Autodesk Inventor part; units mm, degrees
ref_plane "YZ Plane" through (0, 0, 0) normal (1, 0, 0) x (0, 1, 0)
ref_plane "XZ Plane" through (0, 0, 0) normal (0, 1, 0) x (-1, 0, 0)
ref_plane "XY Plane" through (0, 0, 0) normal (0, 0, 1) x (1, 0, 0)
sketch "Sketch1" plane through (0, 0, 0) normal (1, 0, 0) x (0, 1, 0)
  circle A0 centre (0, 0) radius 3
  dimension "d0" = 6
extrude "Extrusion1" add sketch "Sketch1" along normal mid plane 18
sketch "Sketch2" plane through (-9, 0, 0) normal (-1, 0, 0) x (0, 0, 1)
  circle A0 centre (0, 0) radius 4.5
  dimension "d3" = 9
extrude "Extrusion2" add sketch "Sketch2" along normal blind 1
sketch "Sketch3" plane through (9, 0, 0) normal (1, 0, 0) x (0, 0, -1)
  circle A0 centre (0, 0) radius 3.25
  dimension "d6" = 6.5
extrude "Extrusion3" add sketch "Sketch3" along normal blind 1
sketch "Sketch4" plane through (10, 0, 0) normal (1, 0, 0) x (0, 0, -1)
  circle A0 centre (0, 0) radius 3.25
  line L0 (-3.1282, 0.8815) -> (3.1282, 0.8815)
  line L1 (-3.25, 0) -> (3.25, 0)
  line L2 (-3.1282, -0.8815) -> (3.1282, -0.8815)
  arc A1 (-3.1282, 0.8815) -> (-3.1282, -0.8815) centre (0, 0) ccw
  arc A2 (3.1282, -0.8815) -> (3.1282, 0.8815) centre (0, 0) ccw
extrude "Extrusion4" cut sketch "Sketch4" against normal blind 19 contours L1 A0 L0 | A0 L2 L1
fillet "Fillet1" radius 2 2 edges at (10, 3.25, 0) (10, -3.25, 0)
properties part number "OsovinaZaPrednjiKotač_v.1.0"
The model under review builds one solid part; all positions refer to its coordinate system, in mm. A direction names the side the tool comes from. Round coordinates to 2 decimals unless told otherwise and drop trailing zeros. Order: outer loops, then holes, each group sorted by start corner. A loop starts at its lowest first (then second) coordinate and runs counter-clockwise, first axis right, second up. Notation, with made-up numbers: (-40, 53) -> (-5, 53) arc R21 ccw to (-5, 72) -> close; hole circle Ø10 at (54, -9). An arc over 180 degrees is marked (long way). One line per item, written item: value. Start each with the question number.
Q1. Take a section at A-A (x = 5.5). Write out the cut boundary in (y, z), and give its area (3 significant figures).
Q2. Clearance check with flat-ended pins moving along their axes: pin 1 Ø5 at (x, z) = (4.5, 1.5) entering from +Y; pin 2 Ø1.5 at (y, z) = (-2, 1.5) entering from +X; pin 3 Ø1.5 at (x, y) = (3.5, 3.5) entering from +Z. State where each tip first meets the part, or that it passes through.
Q3. Take a section at B-B (y = 4). Write out the cut boundary in (x, z), and give its area (3 significant figures).
Q4. Mouldability with a two-part tool opening along X and no side actions: class faces 4 (the face through (-10, 0, 0)), 5 (the face through (0, -3, 0)), 6 (the face through (0, 3, 0)), 7 (the face through (1, -0.882, 0)) as released by +X, released by -X, zero draft, split by the parting line, or undercut.
Q5. Wall thickness on line 1 (X direction, y = 4, z = 0); line 2 (Y direction, x = 7.75, z = 0.75); line 3 (Y direction, x = -4.5, z = 1.75): over which ranges is each line inside the solid? List them lowest first.
Q6. Machinability: for faces 1 (the face through (-9, 0, 0)), 2 (the face through (1, 0.882, 0)), 3 (the face through (-9.49, -4.46, -0.59)), which of the approach directions +Z, -Z, +X, -X, +Y, -Y give a long, thin tool a straight path to every point of the face, cutting with its end or side? Answer none if there is none.
Reported:
1. outline: (-0.88, -2.87) -> (-0.88, 2.87) arc R3 ccw to start; (0.88, -2.87) arc R3 ccw to (0.88, 2.87) -> close
1. area: 17.9 mm2
2. pin 1: stops at y = 3
2. pin 2: stops at x = 9.99
2. pin 3: stops at z = 1.2
3. outline: (-10, -2.06) -> (-9, -2.06) -> (-9, 2.06) -> (-10, 2.06) -> close
3. area: 4.12 mm2
4. face 4: released by -X
4. face 5: undercut
4. face 6: undercut
4. face 7: zero draft
5. line 1: x = -10 to -9
5. line 2: y = -2.9 to -0.88, 0.88 to 2.9
5. line 3: y = -2.44 to -0.88, 0.88 to 2.44
6. face 1: none
6. face 2: +Z, -Z, +X
6. face 3: +X, -X
